from build123d import *

# Parameters (mm, degrees)
BOX003_W        = 5
BOX003_H        = 20
BOX003_DEPTH    = 15
POCKET004_DEPTH = 5.001
BOX002_W        = 5
BOX002_H        = 20
BOX002_DEPTH    = 15
POCKET003_DEPTH = 5.001
BOX_W           = 80
BOX_H           = 6
BOX_DEPTH       = 30
POCKET002_DEPTH = 6.001
BOX001_W        = 36
BOX001_H        = 37
BOX001_DEPTH    = 9
SKETCH_R        = 11
POCKET_DEPTH    = 7
SKETCH001_R     = 6
POCKET001_DEPTH = 2.001
CHAMFER_SIZE    = 5
FILLET_R        = 10
FILLET001_R     = 10


with BuildPart() as pocket004:
    # Box003 → Box003 (new body)
    with BuildSketch(Plane(origin=(53, -20, 9), x_dir=(1, 0, 0), z_dir=(0, 0, 1))):
        with Locations((2.5, 10)):
            Rectangle(BOX003_W, BOX003_H)
    extrude(amount=BOX003_DEPTH)

    # Sketch005 → Pocket004 (cut, through all)
    with BuildSketch(Plane(origin=(58, -20, 9), x_dir=(0, 1, 0), z_dir=(1, 0, 0))):
        Polygon((0, 0), (20, 15), (0, 15), align=None)
    extrude(amount=-POCKET004_DEPTH, mode=Mode.SUBTRACT)


with BuildPart() as pocket003:
    # Box002 → Box002 (new body)
    with BuildSketch(Plane(origin=(22, -20, 9), x_dir=(1, 0, 0), z_dir=(0, 0, 1))):
        with Locations((2.5, 10)):
            Rectangle(BOX002_W, BOX002_H)
    extrude(amount=BOX002_DEPTH)

    # Sketch004 → Pocket003 (cut, through all)
    with BuildSketch(Plane(origin=(27, -20, 9), x_dir=(0, 1, 0), z_dir=(1, 0, 0))):
        Polygon((20, 15), (0, 0), (0, 15), align=None)
    extrude(amount=-POCKET003_DEPTH, mode=Mode.SUBTRACT)


with BuildPart() as pocket002:
    # Box → Box (new body)
    with BuildSketch(Plane.XY):
        with Locations((40, 3)):
            Rectangle(BOX_W, BOX_H)
    extrude(amount=BOX_DEPTH)

    # Sketch003 → Pocket002 (cut, through all)
    with BuildSketch(Plane.XZ):
        with BuildLine():
            ThreePointArc((15.75, 22), (12.5, 25.25), (9.25, 22))
            Line((9.25, 22), (9.25, 8))
            ThreePointArc((9.25, 8), (12.5, 4.75), (15.75, 8))
            Line((15.75, 22), (15.75, 8))
        make_face()
        with BuildLine():
            ThreePointArc((70.75, 22), (67.5, 25.25), (64.25, 22))
            Line((64.25, 22), (64.25, 8))
            ThreePointArc((64.25, 8), (67.5, 4.75), (70.75, 8))
            Line((70.75, 22), (70.75, 8))
        make_face()
    extrude(amount=-POCKET002_DEPTH, mode=Mode.SUBTRACT)


with BuildPart() as fillet001:
    # Box001 → Box001 (new body)
    with BuildSketch(Plane(origin=(22, -37, 0), x_dir=(1, 0, 0), z_dir=(0, 0, 1))):
        with Locations((18, 18.5)):
            Rectangle(BOX001_W, BOX001_H)
    extrude(amount=BOX001_DEPTH)

    # Sketch → Pocket (cut)
    with BuildSketch(Plane(origin=(22, -37, 9), x_dir=(1, 0, 0), z_dir=(0, 0, 1))):
        with Locations((18, 15)):
            Circle(SKETCH_R)
    extrude(amount=-POCKET_DEPTH, mode=Mode.SUBTRACT)

    # Sketch001 → Pocket001 (cut, through all)
    with BuildSketch(Plane(origin=(22, -37, 2), x_dir=(1, 0, 0), z_dir=(0, 0, 1))):
        with Locations((18, 15)):
            Circle(SKETCH001_R)
    extrude(amount=-POCKET001_DEPTH, mode=Mode.SUBTRACT)

    # Fusion: union Pocket004, Pocket003, Pocket002
    add(pocket004.part)
    add(pocket003.part)
    add(pocket002.part)

    # Chamfer
    chamfer_edges = [fillet001.edges().sort_by_distance(p)[0] for p in [
        (40, 0, 9),
    ]]
    chamfer(chamfer_edges, length=CHAMFER_SIZE)

    # Fillet
    fillet_edges = [fillet001.edges().sort_by_distance(p)[0] for p in [
        (58, -37, 4.5),
    ]]
    fillet(fillet_edges, radius=FILLET_R)

    # Fillet001
    fillet001_edges = [fillet001.edges().sort_by_distance(p)[0] for p in [
        (22, -37, 4.5),
    ]]
    fillet(fillet001_edges, radius=FILLET001_R)


solid = fillet001.part
Could you check a few things on this model? Use its own coordinates, in mm. A direction names the side the tool comes from. Give positions to 0.01 mm unless a question says otherwise; leave off trailing zeros. Order: outer loops, then holes, each group sorted by start corner. A loop starts at its lowest first (then second) coordinate and runs counter-clockwise, first axis right, second up. Notation, with made-up numbers: (72.5, -30.75) -> (107.5, -30.75) arc R26 cw to (107.5, -5.75) -> close; hole circle Ø6 at (34, 20.5). An arc over 180 degrees is marked (long way). Answer in a Markdown table with one row per item. Add a question column.
Item 1: Imagine slicing it at A-A (x = 12.5). List the corners of the cut face in (y, z) for me.
Item 2: Imagine slicing it at D-D (x = 40). List the corners of the cut face in (y, z) for me.
Item 3: Please list where these lines run through material, in increasing order: probe 1 along Y at (x, z) = (40, 0.9); probe 2 along Y at (x, z) = (40, 5); probe 3 along Z at (x, y) = (46, -28.5).
Item 4: Imagine slicing it at C-C (z = 20.75). List the corners of the cut face in (x, y) for me, and give its area (3 significant figures).
Item 5: Imagine slicing it at B-B (y = -22). List the corners of the cut face in (x, z) for me.
Item 6: We'd pull the mould along X, two halves only. Please class faces 4 (the flat face through (39, 6, 15)), 5 (the cylindrical face through (12.43, 2.96, 4.75)), 6 (the cylindrical face through (25.01, -34.15, 4.56)), 7 (the flat face through (39, 0, 18)): pulls with the +X half, pulls with the -X half, needs draft (parallel to the pull), parting line crosses it, or undercut.
Item 7: For faces 1 (the flat face through (45, -27, 2)), 2 (the flat face through (64.25, 3, 15)), 3 (the flat face through (40, -3, 11)), which set-ups out of +Z, -Z, +X, -X, +Y, -Y let a thin tool reach every point of the face, with its end or its side?
Item 8: I'm going to push flat-ended pins straight in: P1, Ø24, axis at x = 39.5, y = -27, coming from the +Z side; P2, Ø9.5, axis at x = 40, y = -22, coming from the -Z side; P3, Ø6, axis at x = 15.5, z = 21.5, coming from the -Y side; P4, Ø12, axis at y = -11, z = 15.5, coming from the -X side. Where does each tip first touch, or does it pass through?
Result:
| question | item | result |
|---|---|---|
| 1 | outline | (0, 0) -> (6, 0) -> (6, 4.75) -> (0, 4.75) -> close; (0, 25.25) -> (6, 25.25) -> (6, 30) -> (0, 30) -> close |
| 2 | outline | (-37, 0) -> (-28, 0) -> (-28, 2) -> (-33, 2) -> (-33, 9) -> (-37, 9) -> close; (-16, 0) -> (6, 0) -> (6, 30) -> (0, 30) -> (0, 14) -> (-5, 9) -> (-11, 9) -> (-11, 2) -> (-16, 2) -> close |
| 3 | probe 1 | -37 to -28, -16 to 6 |
| 3 | probe 2 | -37 to -33, -11 to 6 |
| 3 | probe 3 | 0 to 2 |
| 4 | outline | (0, 0) -> (9.25, 0) -> (9.25, 6) -> (0, 6) -> close; (15.75, 0) -> (22, 0) -> (22, -4.33) -> (27, -4.33) -> (27, 0) -> (53, 0) -> (53, -4.33) -> (58, -4.33) -> (58, 0) -> (64.25, 0) -> (64.25, 6) -> (15.75, 6) -> close; (70.75, 0) -> (80, 0) -> (80, 6) -> (70.75, 6) -> close |
| 4 | area | 445 mm2 |
| 5 | outline | (22, 0) -> (34, 0) -> (34, 2) -> (29, 2) -> (29, 9) -> (22, 9) -> close; (46, 0) -> (58, 0) -> (58, 9) -> (51, 9) -> (51, 2) -> (46, 2) -> close |
| 6 | face 4 | needs draft |
| 6 | face 5 | undercut |
| 6 | face 6 | pulls with the -X half |
| 6 | face 7 | undercut |
| 7 | face 1 | +Z |
| 7 | face 2 | +Y, -Y |
| 7 | face 3 | +Z, -Y |
| 8 | P1 | z = 9 |
| 8 | P2 | through |
| 8 | P3 | y = 0 |
| 8 | P4 | x = 22 |
